Design review of the part built by this model. Coordinates are the model's own, in mm. Face numbers are marked on the shaded views. A direction names the side the tool comes from. Round coordinates to 2 decimals unless told otherwise and drop trailing zeros. Loops run counter-clockwise (first coordinate to the right, second up) from the corner with the lowest first, then second, coordinate; pieces in that order, holes last. Notation, with made-up numbers: (70, -21.75) - (124, -21.75) arc R21 ccw to (124, 9.25) - close; hole circle Ø7 at (47.5, 37). An arc over 180 degrees is marked (long way). Answer as CSV lines item,"result". Start each with the question number.
(1) Consider section C-C (z = 0). Give the boundary of the cut face in (x, y).
(2) Consider section A-A (y = 510). Give the boundary of the cut face in (x, z).
(3) Consider section B-B (x = 0). Give the boundary of the cut face in (y, z), and give its area (3 significant figures).
(4) For P1, Ø1, axis at x = -38, z = 32, coming from the +Y side; P2, Ø8, axis at y = 157, z = 12, coming from the +X side; P3, Ø1, axis at x = 43.5, z = 20.5, coming from the -Y side; P4, Ø2, axis at x = 1, z = -0.5, coming from the -Y side, all flat-tipped, find the tip position at first contact; note any pin that passes through.
(5) Consider section D-D (y = 228). Give the boundary of the cut face in (x, z), and give its area (3 significant figures).
(6) For the marked faces 1, 2, 3 and 4, list the 3-axis set-ups (+Z, -Z, +X, -X, +Y, -Y) from which the entire face can be reached by the end or side of a thin tool; tool diameter is ignored.
(7) Wall thickness on L1, parallel to X at y = 468.5, z = 32.5; L2, parallel to Y at x = 27, z = 5; L3, parallel to Y at x = 27, z = -27.5: over which ranges is each line inside the solid? List them lowest first.
(8) Mouldability with a two-part tool opening along Y and no side actions: class the marked faces 5, 6 and 7 as released by +Y, released by -Y, zero draft, split by the parting line, or undercut.
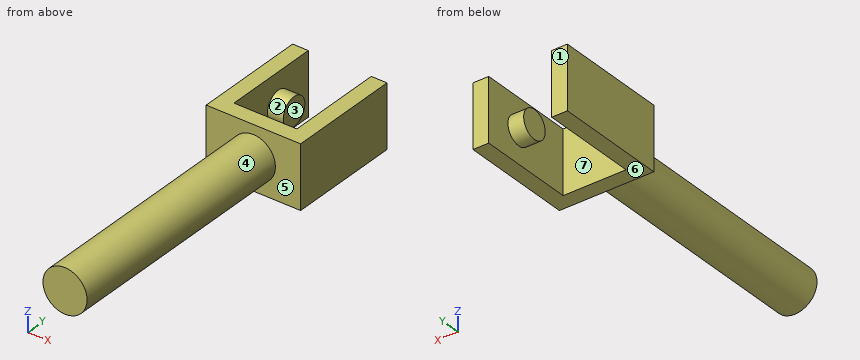
from build123d import *

# Parameters (mm, degrees)
SKETCH1_R           = 35
BOSS_EXTRUDE1_DEPTH = 392.5
SKETCH2_W           = 150
SKETCH2_H           = 100
BOSS_EXTRUDE2_DEPTH = 180
SKETCH3_W           = 100
SKETCH3_H           = 125
CUT_EXTRUDE1_DEPTH  = 150
SKETCH4_R           = 22.5
BOSS_EXTRUDE3_DEPTH = 25
BOSS_EXTRUDE4_START = 25
SKETCH5_R           = 22.5
BOSS_EXTRUDE4_DEPTH = 25
SKETCH6_W           = 100
SKETCH6_H           = 30
CUT_EXTRUDE2_DEPTH  = 586.987414541


with BuildPart() as part:
    # Sketch1 → Boss-Extrude1 (new body)
    with BuildSketch(Plane(origin=(0, 0, 0), x_dir=(1, 0, 0), z_dir=(0, 1, 0))):
        with Locations(Location((0, 0, 0), (0, 0, 270))):
            Circle(SKETCH1_R)
    extrude(amount=BOSS_EXTRUDE1_DEPTH)

    # Sketch2 → Boss-Extrude2 (add)
    with BuildSketch(Plane(origin=(0, 392.5, 0), x_dir=(1, 0, 0), z_dir=(0, 1, 0))):
        Rectangle(SKETCH2_W, SKETCH2_H)
    extrude(amount=BOSS_EXTRUDE2_DEPTH)

    # Sketch3 → Cut-Extrude1 (cut)
    with BuildSketch(Plane.XY.offset(50)):
        with Locations((0, 510)):
            Rectangle(SKETCH3_W, SKETCH3_H)
    extrude(amount=-CUT_EXTRUDE1_DEPTH, mode=Mode.SUBTRACT)

    # Sketch4 → Boss-Extrude3 (add)
    with BuildSketch(Plane.ZY.offset(-50)):
        with Locations(Location((0, 510, 0), (0, 0, 90))):
            Circle(SKETCH4_R)
    extrude(amount=BOSS_EXTRUDE3_DEPTH)

    # Sketch5 → Boss-Extrude4 (add)
    with BuildSketch(Plane(origin=(-50, 0, 0), x_dir=(0, 0, -1), z_dir=(1, 0, 0)).offset(BOSS_EXTRUDE4_START)):
        with Locations(Location((0, 510, 0), (0, 0, 90))):
            Circle(SKETCH5_R)
    extrude(amount=-BOSS_EXTRUDE4_DEPTH)

    # Sketch6 → Cut-Extrude2 (cut, through all)
    with BuildSketch(Plane.XY.offset(50)):
        with Locations((0, 432.5)):
            Rectangle(SKETCH6_W, SKETCH6_H)
    extrude(amount=-CUT_EXTRUDE2_DEPTH, mode=Mode.SUBTRACT)


solid = part.part
Determined:
1,outline,"(-75, 392.5) - (-35, 392.5) - (-35, 0) - (35, 0) - (35, 392.5) - (75, 392.5) - (75, 572.5) - (50, 572.5) - (50, 532.5) - (25, 532.5) - (25, 487.5) - (50, 487.5) - (50, 417.5) - (-50, 417.5) - (-50, 487.5) - (-25, 487.5) - (-25, 532.5) - (-50, 532.5) - (-50, 572.5) - (-75, 572.5) - close"
2,outline,"(-75, -50) - (-50, -50) - (-50, -22.5) - (-25, -22.5) - (-25, 22.5) - (-50, 22.5) - (-50, 50) - (-75, 50) - close; (25, -22.5) - (50, -22.5) - (50, -50) - (75, -50) - (75, 50) - (50, 50) - (50, 22.5) - (25, 22.5) - close"
3,outline,"(0, -35) - (392.5, -35) - (392.5, -50) - (417.5, -50) - (417.5, 50) - (392.5, 50) - (392.5, 35) - (0, 35) - close"
3,area,"30,000 mm^2"
4,P1,"stops at y = 417.5"
4,P2,"stops at x = 34.07"
4,P3,"stops at y = 392.5"
4,P4,"stops at y = 0"
5,outline,"circle Ø70 at (0, 0)"
5,area,"3,850 mm^2"
6,face 1,"+Z, -Z, +X, -X, +Y"
6,face 2,"none"
6,face 3,"+Z, -Z, +Y"
6,face 4,"-Y"
7,L1,"x = -75 to -50, 50 to 75"
7,L2,"y = 0 to 417.5, 488.06 to 531.94"
7,L3,"y = 392.5 to 417.5"
8,face 5,"released by -Y"
8,face 6,"zero draft"
8,face 7,"undercut"
